Read the model definition and answer for the solid it produces. Units are mm, in the model's axes. A direction names the side the tool comes from. Coordinates: 2 decimals unless noted, no trailing zeros. Write each loop counter-clockwise with the first axis right and the second up, starting at its lowest first coordinate (ties: lowest second). Pieces come first, ordered by that corner, then holes. Notation, with made-up numbers: M 63,4 L 108,4 A25 cw 108,39 Z; hole C 37,74.25 d4. An arc over 180 degrees is marked long. Write item = value, one per line.
from build123d import *

# Parameters (mm, degrees)
SKETCH1_R           = 1.75
BOSS_EXTRUDE1_DEPTH = 2
SKETCH2_R           = 2.25
BOSS_EXTRUDE2_DEPTH = 1
CUT_EXTRUDE1_DEPTH  = 1


with BuildPart() as part:
    # Sketch1 → Boss-Extrude1 (new, symmetric)
    with BuildSketch(Plane(origin=(0, 0, 0), x_dir=(1, 0, 0), z_dir=(0, 1, 0))):
        with Locations(Location((0, 0, 0), (0, 0, 270))):
            Circle(SKETCH1_R)
    extrude(amount=BOSS_EXTRUDE1_DEPTH, both=True)

    # Sketch2 → Boss-Extrude2 (add)
    with BuildSketch(Plane(origin=(0, 2, 0), x_dir=(1, 0, 0), z_dir=(0, 1, 0))):
        with Locations(Location((0, 0, 0), (0, 0, 270))):
            Circle(SKETCH2_R)
    extrude(amount=BOSS_EXTRUDE2_DEPTH)

    # Sketch3 → Cut-Extrude1 (cut)
    with BuildSketch(Plane(origin=(0, 3, 0), x_dir=(1, 0, 0), z_dir=(0, 1, 0))):
        Polygon((1.154700538, 0), (0.577350269, 1), (-0.577350269, 1), (-1.154700538, 0), (-0.577350269, -1), (0.577350269, -1), align=None)
    extrude(amount=-CUT_EXTRUDE1_DEPTH, mode=Mode.SUBTRACT)


solid = part.part
Item 1: Find section D-D (y = -1.25). Determine the outline of the cut face in (x, z).
Worked answers:
outline = C 0,0 d3.5
Item 2: Find section A-A (y = 2.35). Determine the outline of the cut face in (x, z), and give its area (3 significant figures).
Worked answers:
outline = C 0,0 d4.5; hole M -1.15,0 L -0.58,-1 L 0.58,-1 L 1.15,0 L 0.58,1 L -0.58,1 Z
area = 12.4 mm²
Item 3: For a pull along Y with two mould halves and no side action, classify faces 1 (the face through (0, 2.5, 1)), 2 (the face through (0, 2, 0)), 3 (the face through (0, -2, 0)) as released by +Y, released by -Y, zero draft, split by the parting line, or undercut.
Worked answers:
face_1 = zero draft
face_2 = released by +Y
face_3 = released by -Y
Item 4: Consider line 1 along Y through (x, z) = (-0.6, -0.6); line 2 along Y through (x, z) = (-1.5, 1.55); line 3 along X through (y, z) = (-0.7, 0.25). Determine where each line is inside the solid, lowest interval first. Write a range as from..to.
Worked answers:
line_1 = -2..2
line_2 = 2..3
line_3 = -1.73..1.73
Item 5: Which of the six approach directions +Z, -Z, +X, -X, +Y, -Y give full straight-line access (tool end or side, diameter ignored) to faces 4 (the face through (0.87, 2.51, -0.49)), 5 (the face through (0.676, 2.493, 2.146)), 6 (the face through (-1.71, 0.03, -0.38))?
Worked answers:
face_4 = +Y
face_5 = +Y, -Y
face_6 = -Y
Item 6: Find section C-C (x = -1.5). Determine the outline of the cut face in (y, z).
Worked answers:
outline = M -2,-0.9 L 2,-0.9 L 2,-1.68 L 3,-1.68 L 3,1.68 L 2,1.68 L 2,0.9 L -2,0.9 Z
Item 7: Find section B-B (z = 1.1). Determine the outline of the cut face in (x, y).
Worked answers:
outline = M -1.96,2 L -1.36,2 L -1.36,-2 L 1.36,-2 L 1.36,2 L 1.96,2 L 1.96,3 L -1.96,3 Z
